Check sheet for the drawn part. Datum: minimum x, y, z corner. Units: mm. Round coordinates to 2 decimals unless told otherwise and drop trailing zeros. Write each loop counter-clockwise with the first axis right and the second up, starting at its lowest first coordinate (ties: lowest second). Pieces come first, ordered by that corner, then holes.
Item 1: Cross-section at D-D on x = 4. Enter the section's corners in (y, z), plus the area to 3 significant figures.
Item 2: Go/stop test with flat-tipped pins: pin 1 Ø1 at (x, y) = (6.5, 3) entering from -Z; pin 2 Ø1.5 at (x, z) = (2.5, 26.5) entering from +Y. Record where each tip stops, or that it passes through.
Item 3: Material ranges on line 1 (Z direction, x = 3.75, y = 6.5); line 2 (Y direction, x = 6.5, z = 10.75); line 3 (X direction, y = 4.25, z = 10.5), recorded low to high.
Item 4: Cross-section at C-C on z = 25. Enter the section's corners in (x, y).
Item 5: Cross-section at A-A on y = 4. Enter the section's corners in (x, z) (3 decimals), plus the area to 3 significant figures.
Item 6: Cross-section at B-B on x = 2.25. Enter the section's corners in (y, z) (3 decimals), plus the area to 3 significant figures.
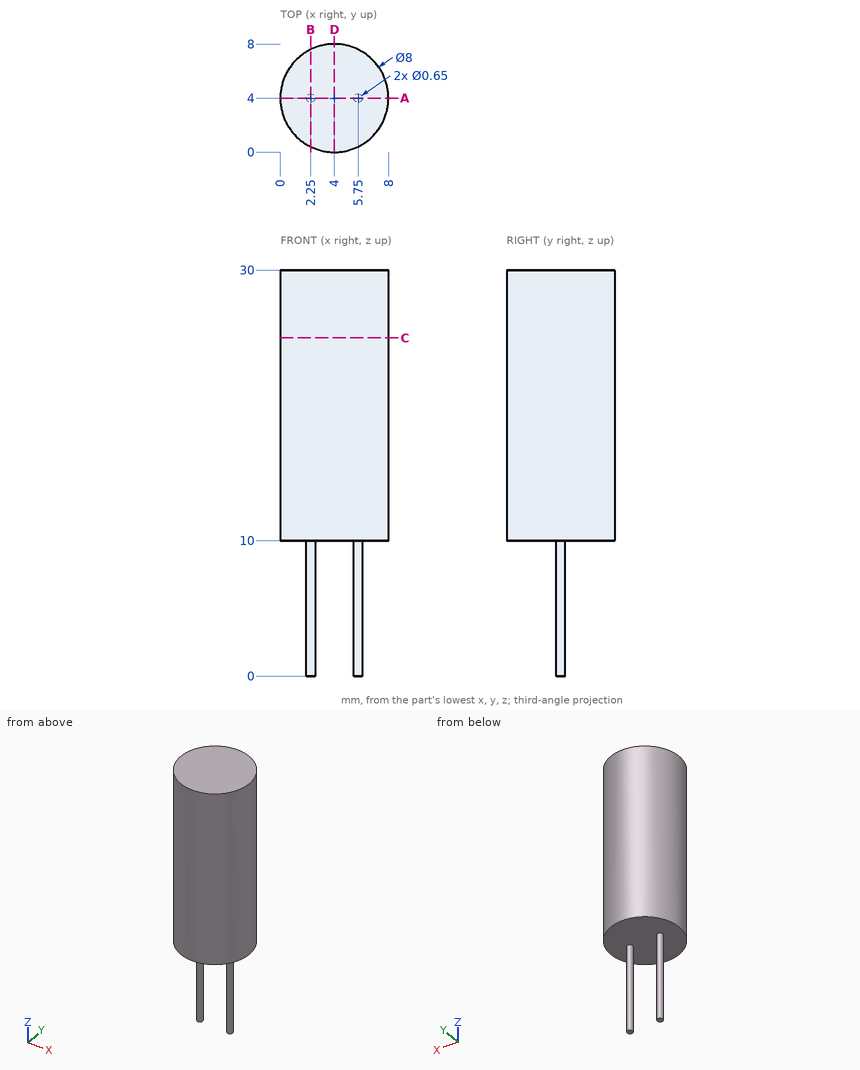
Response values:
1. outline: (0, 10) - (8, 10) - (8, 30) - (0, 30) - close
1. area: 160 mm2
2. pin 1: stops at z = 10
2. pin 2: stops at y = 7.93
3. line 1: z = 10 to 30
3. line 2: y = 0.88 to 7.12
3. line 3: x = 0.01 to 7.99
4. outline: circle Ø8 at (4, 4)
5. outline: (0, 10) - (1.925, 10) - (1.925, 0) - (2.575, 0) - (2.575, 10) - (5.425, 10) - (5.425, 0) - (6.075, 0) - (6.075, 10) - (8, 10) - (8, 30) - (0, 30) - close
5. area: 173 mm2
6. outline: (0.403, 10) - (3.675, 10) - (3.675, 0) - (4.325, 0) - (4.325, 10) - (7.597, 10) - (7.597, 30) - (0.403, 30) - close
6. area: 150 mm2
